from build123d import *

# Parameters (mm, degrees)
SKETCH1_W           = 308
SKETCH1_H           = 50
SKETCH1_R           = 6
SKETCH1_R_2         = 1.2
BOSS_EXTRUDE1_DEPTH = 8
SKETCH2_W           = 8
SKETCH2_H           = 20
BOSS_EXTRUDE2_DEPTH = 8


with BuildPart() as part:
    # Sketch1 → Boss-Extrude1 (new body)
    with BuildSketch(Plane(origin=(0, 0, 0), x_dir=(1, 0, 0), z_dir=(0, 1, 0))):
        with Locations((154, 25)):
            Rectangle(SKETCH1_W, SKETCH1_H)
        with Locations((75, 25)):
            Circle(SKETCH1_R, mode=Mode.SUBTRACT)
        with Locations((59.5, 40.5)):
            Circle(SKETCH1_R_2, mode=Mode.SUBTRACT)
        with Locations((90.5, 40.5)):
            Circle(SKETCH1_R_2, mode=Mode.SUBTRACT)
        with Locations((59.5, 9.5)):
            Circle(SKETCH1_R_2, mode=Mode.SUBTRACT)
        with Locations((90.5, 9.5)):
            Circle(SKETCH1_R_2, mode=Mode.SUBTRACT)
        with Locations((217.5, 9.5)):
            Circle(SKETCH1_R_2, mode=Mode.SUBTRACT)
        with Locations((248.5, 9.5)):
            Circle(SKETCH1_R_2, mode=Mode.SUBTRACT)
        with Locations((217.5, 40.5)):
            Circle(SKETCH1_R_2, mode=Mode.SUBTRACT)
        with Locations((233, 25)):
            Circle(SKETCH1_R, mode=Mode.SUBTRACT)
        with Locations((248.5, 40.5)):
            Circle(SKETCH1_R_2, mode=Mode.SUBTRACT)
    extrude(amount=BOSS_EXTRUDE1_DEPTH)

    # Sketch2 → Boss-Extrude2 (add)
    with BuildSketch(Plane(origin=(0, 8, 0), x_dir=(-1, 0, 0), z_dir=(0, 1, 0))):
        with Locations((4, -25)):
            Rectangle(SKETCH2_W, SKETCH2_H)
        with Locations((-312, -25)):
            Rectangle(SKETCH2_W, SKETCH2_H)
    extrude(amount=-BOSS_EXTRUDE2_DEPTH)


solid = part.part
Work out the finished part from the listing and answer in its coordinate system (mm). A direction names the side the tool comes from. Coordinates: 2 decimals unless noted, no trailing zeros. Loops run counter-clockwise (first coordinate to the right, second up) from the corner with the lowest first, then second, coordinate; pieces in that order, holes last. Notation, with made-up numbers: M 76.25,-40 L 103.25,-40 A23 cw 103.25,-21 Z; hole C 61.5,46 d1. An arc over 180 degrees is marked long. Answer in a Markdown table with one row per item. Add a question column.
1. Flat-ended cylindrical pins translate along their axes: P1, Ø4, axis at x = 59.5, z = -9.5, coming from the +Y side; P2, Ø2.5, axis at y = 5.5, z = -11, coming from the -X side; P3, Ø4, axis at x = -6, y = 3, coming from the -Z side; P4, Ø2.5, axis at y = 3, z = -45, coming from the +X side. Find the tip coordinate at first contact, or state that the pin passes through.
2. The mould has two halves that part along X. Classify faces 1 (the flat face through (0, 4, -42)), 2 (the cylindrical face through (238.723, 3.944, -26.802)), 3 (the cylindrical face through (69, 4, -25)), 4 (the flat face through (312, 4, -35)): pulls with the +X half, pulls with the -X half, needs draft (parallel to the pull), parting line crosses it, or undercut.
3. Find section A-A, the plane y = 5.25. State how many separate pieces and enclosed holes the cut face has, then the cut area to 3 significant figures.
4. A tool of negligible diameter and unlimited length cuts with its end or side. For faces 5 (the flat face through (-4, 4, -15)), 6 (the flat face through (308, 4, -42)), 7 (the flat face through (308, 4, -7)), 8 (the flat face through (-8, 4, -25)), 9 (the flat face through (-4, 4, -35)), from which of +Z, -Z, +X, -X, +Y, -Y can it reach the whole face along a straight path? Write none if from no direction.
5. Consider L1, parallel to X at y = 3, z = -40.5; L2, parallel to Z at x = 90.5, y = 5.5; L3, parallel to X at y = 1.25, z = -27. Determine where each line is inside the solid, lowest interval first.
6. Find section B-B, the plane x = 233. Write down the section's boundary in (y, z), then the cut area to 3 significant figures.
Reported:
| question | item | result |
|---|---|---|
| 1 | P1 | stops at y = 8 |
| 1 | P2 | stops at x = 0 |
| 1 | P3 | stops at z = -35 |
| 1 | P4 | stops at x = 308 |
| 2 | face 1 | pulls with the -X half |
| 2 | face 2 | undercut |
| 2 | face 3 | undercut |
| 2 | face 4 | needs draft |
| 3 | separate pieces | 1 |
| 3 | enclosed holes | 10 |
| 3 | area | 15,500 mm^2 |
| 4 | face 5 | +Z, -X, +Y, -Y |
| 4 | face 6 | -Z, +X, +Y, -Y |
| 4 | face 7 | +Z, +X, +Y, -Y |
| 4 | face 8 | +Z, -Z, -X, +Y, -Y |
| 4 | face 9 | -Z, -X, +Y, -Y |
| 5 | L1 | x = 0 to 58.3, 60.7 to 89.3, 91.7 to 216.3, 218.7 to 247.3, 249.7 to 308 |
| 5 | L2 | z = -50 to -41.7, -39.3 to -10.7, -8.3 to 0 |
| 5 | L3 | x = -8 to 69.34, 80.66 to 227.34, 238.66 to 316 |
| 6 | outline | M 0,-50 L 8,-50 L 8,-31 L 0,-31 Z; M 0,-19 L 8,-19 L 8,0 L 0,0 Z |
| 6 | area | 304 mm^2 |
